Check sheet for the modelled part. Datum: model origin and axes. Units: mm. Give positions to 0.01 mm unless a question says otherwise; leave off trailing zeros. Order: outer loops, then holes, each group sorted by start corner. A loop starts at its lowest first (then second) coordinate and runs counter-clockwise, first axis right, second up. Notation, with made-up numbers: M -38.75,64 L 8.25,64 A25 ccw 8.25,88 Z; hole C 13.5,31 d4. An arc over 180 degrees is marked long. Answer in a Markdown table with one row per item. Add a question column.
from build123d import *

# Parameters (mm, degrees)
SKETCH_1_R          = 1.5
SKETCH_1_W          = 17
SKETCH_1_H          = 11
EXTRUDE_1_DEPTH     = 1
CUT_EXTRUDE_1_DEPTH = 109.245092268


with BuildPart() as part:
    # Эскиз1 → Бобышка-Вытянуть1 (new body)
    with BuildSketch(Plane(origin=(0, 0, 0), x_dir=(-1, 0, 0), z_dir=(0, 0, 1))):
        Polygon((47.5, 21), (15, 21), (15, 48), (-50, 48), (-50, -48), (15, -48), (15, -21), (47.5, -21), align=None)
        with Locations(Location((20.8, -15.6, 0), (0, 0, 180))):
            Circle(SKETCH_1_R, mode=Mode.SUBTRACT)
        with Locations(Location((20.8, -5.2, 0), (0, 0, 180))):
            Circle(SKETCH_1_R, mode=Mode.SUBTRACT)
        with Locations(Location((20.8, 5.2, 0), (0, 0, 180))):
            Circle(SKETCH_1_R, mode=Mode.SUBTRACT)
        with Locations(Location((20.8, 15.6, 0), (0, 0, 180))):
            Circle(SKETCH_1_R, mode=Mode.SUBTRACT)
        with Locations(Location((44.2, -15.6, 0), (0, 0, 180))):
            Circle(SKETCH_1_R, mode=Mode.SUBTRACT)
        with Locations(Location((44.2, -5.2, 0), (0, 0, 180))):
            Circle(SKETCH_1_R, mode=Mode.SUBTRACT)
        with Locations(Location((44.2, 5.2, 0), (0, 0, 180))):
            Circle(SKETCH_1_R, mode=Mode.SUBTRACT)
        with Locations(Location((44.2, 15.6, 0), (0, 0, 180))):
            Circle(SKETCH_1_R, mode=Mode.SUBTRACT)
        with Locations(Location((9.763297689, -30.5, 0), (0, 0, 180))):
            Circle(SKETCH_1_R, mode=Mode.SUBTRACT)
        with Locations(Location((9.763297689, 30.5, 0), (0, 0, 180))):
            Circle(SKETCH_1_R, mode=Mode.SUBTRACT)
        with Locations(Location((-37.855493079, -36, 0), (0, 0, 180))):
            Circle(SKETCH_1_R, mode=Mode.SUBTRACT)
        with Locations(Location((-37.855493079, 36, 0), (0, 0, 180))):
            Circle(SKETCH_1_R, mode=Mode.SUBTRACT)
        with Locations((-16.751430991, 34.5)):
            Rectangle(SKETCH_1_W, SKETCH_1_H, mode=Mode.SUBTRACT)
        with Locations((-16.751430991, -34.5)):
            Rectangle(SKETCH_1_W, SKETCH_1_H, mode=Mode.SUBTRACT)
    extrude(amount=EXTRUDE_1_DEPTH)

    # Эскиз2 → Вырез-Вытянуть1 (cut, through all)
    with BuildSketch(Plane(origin=(0, 48, 0), x_dir=(1, 0, 0), z_dir=(0, 1, 0))):
        Polygon((47.855493079, -1), (50, 0), (50, -1), align=None)
    extrude(amount=-CUT_EXTRUDE_1_DEPTH, mode=Mode.SUBTRACT)


solid = part.part
Q1. Thickness scan on probe 1 along Y at (x, z) = (-9.5, 0.1); probe 2 along Y at (x, z) = (10, 0.7); probe 3 along Y at (x, z) = (-44.2, 0.7). Record the ranges inside material, lowest first.
Q2. Draft check along Y on faces 1 (the cylindrical face through (-20.995, 17.087, 0.493)), 2 (the flat face through (48.91, 0.67, 0.51)), 3 (the cylindrical face through (-42.77, -15.15, 0.49)). Enter one of: pulls with the +Y half, pulls with the -Y half, needs draft (parallel to the pull), parting line crosses it, or undercut.
Q3. Cross-section at C-C (z = 0.8). State how many separate pieces and enclosed holes the cut face has, and give its area (3 significant figures).
Q4. Cross-section at D-D (y = 15.6). Record the boundary of the cut face in (x, z).
Q5. Go/stop test with flat-tipped pins: pin 1 (0.5 mm diameter, centred on y = 33.5, z = 0.5, fed in from -X); pin 2 (0.5 mm diameter, centred on y = -33, z = 0.5, fed in from +X); pin 3 (0.5 mm diameter, centred on x = -28.5, z = 0.5, fed in from +Y). Record where each tip stops, or that it passes through.
Q6. Cross-section at A-A (y = -30.5). Record the boundary of the cut face in (x, z).
Q7. Cross-section at B-B (x = -20.8). Record the boundary of the cut face in (y, z).
Values follow:
| question | item | result |
|---|---|---|
| 1 | probe 1 | -48 to -31.98, -29.02 to 29.02, 31.98 to 48 |
| 1 | probe 2 | -48 to -40, -29 to 29, 40 to 48 |
| 1 | probe 3 | -21 to -17.1, -14.1 to -6.7, -3.7 to 3.7, 6.7 to 14.1, 17.1 to 21 |
| 2 | face 1 | undercut |
| 2 | face 2 | needs draft |
| 2 | face 3 | undercut |
| 3 | separate pieces | 1 |
| 3 | enclosed holes | 14 |
| 3 | area | 6,980 mm² |
| 4 | outline | M -47.5,0 L -45.7,0 L -45.7,1 L -47.5,1 Z; M -42.7,0 L -22.3,0 L -22.3,1 L -42.7,1 Z; M -19.3,0 L 50,0 L 47.86,1 L -19.3,1 Z |
| 5 | pin 1 | x = -15 |
| 5 | pin 2 | x = 49.46 |
| 5 | pin 3 | y = 21 |
| 6 | outline | M -15,0 L -11.26,0 L -11.26,1 L -15,1 Z; M -8.26,0 L 8.25,0 L 8.25,1 L -8.26,1 Z; M 25.25,0 L 50,0 L 47.86,1 L 25.25,1 Z |
| 7 | outline | M -21,0 L -17.1,0 L -17.1,1 L -21,1 Z; M -14.1,0 L -6.7,0 L -6.7,1 L -14.1,1 Z; M -3.7,0 L 3.7,0 L 3.7,1 L -3.7,1 Z; M 6.7,0 L 14.1,0 L 14.1,1 L 6.7,1 Z; M 17.1,0 L 21,0 L 21,1 L 17.1,1 Z |
